Input: dimensioned drawing with shaded views. Units: mm. Origin: part minimum x, y, z. Coordinates: 2 decimals unless noted, no trailing zeros. Order: outer loops, then holes, each group sorted by start corner. A loop starts at its lowest first (then second) coordinate and runs counter-clockwise, first axis right, second up.
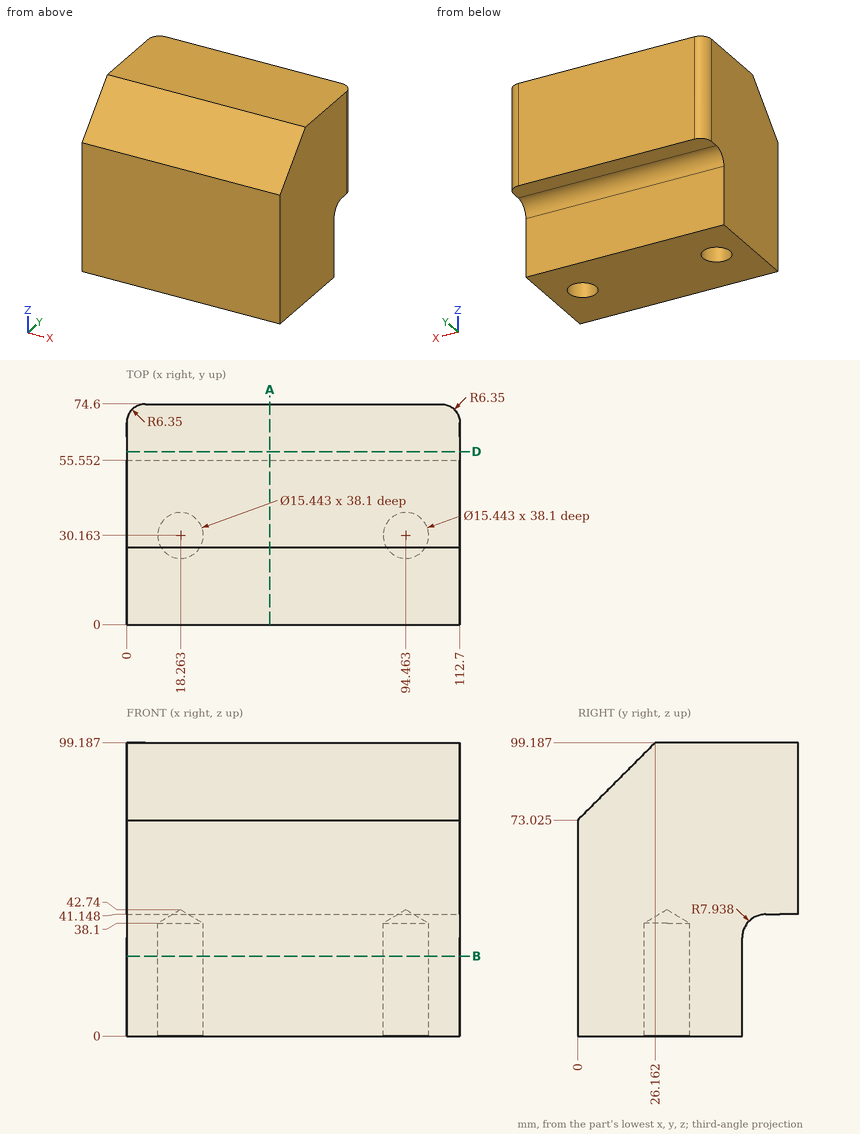
1. Section query D-D on y = 58.5. Return loops of the section in (x, z).
Findings:
outline: (0, 39.38) - (112.7, 39.38) - (112.7, 99.19) - (0, 99.19) - close
2. Section query B-B on z = 27. Return loops of the section in (x, y) (1 decimal), plus the area to 3 significant figures.
Findings:
outline: (0, 0) - (112.7, 0) - (112.7, 55.6) - (0, 55.6) - close; hole circle Ø15.4 at (18.3, 30.2); hole circle Ø15.4 at (94.5, 30.2)
area: 5,890 mm2
3. Ray query, line 1 (Y direction, x = 18, z = 28.5) (1 decimal); line 2 (Y direction, x = 29.5, z = 23) (1 decimal); line 3 (Y direction, x = 12.5, z = 36) (1 decimal). Return the intervals inside material, ascending.
Findings:
line 1: y = 0 to 22.4, 37.9 to 55.6
line 2: y = 0 to 55.6
line 3: y = 0 to 25, 35.3 to 56.1
4. Section query A-A on x = 48.5. Return loops of the section in (y, z) (1 decimal).
Findings:
outline: (0, 0) - (55.6, 0) - (55.6, 33.2) arc R7.9 cw to (63.5, 41.1) - (74.6, 41.1) - (74.6, 99.2) - (26.2, 99.2) - (0, 73) - close
5. Pin query (flat end, axial travel): P1, Ø12.5, axis at x = 94.46, y = 30.16, coming from the -Z side; P2, Ø8, axis at x = 78.5, y = 20, coming from the +Z side (1 decimal); P3, Ø1, axis at x = 88, z = 24, coming from the +Y side (1 decimal). Return the tip coordinate at first contact, or that it passes through.
Findings:
P1: stops at z = 38.98
P2: stops at z = 97
P3: stops at y = 55.6
